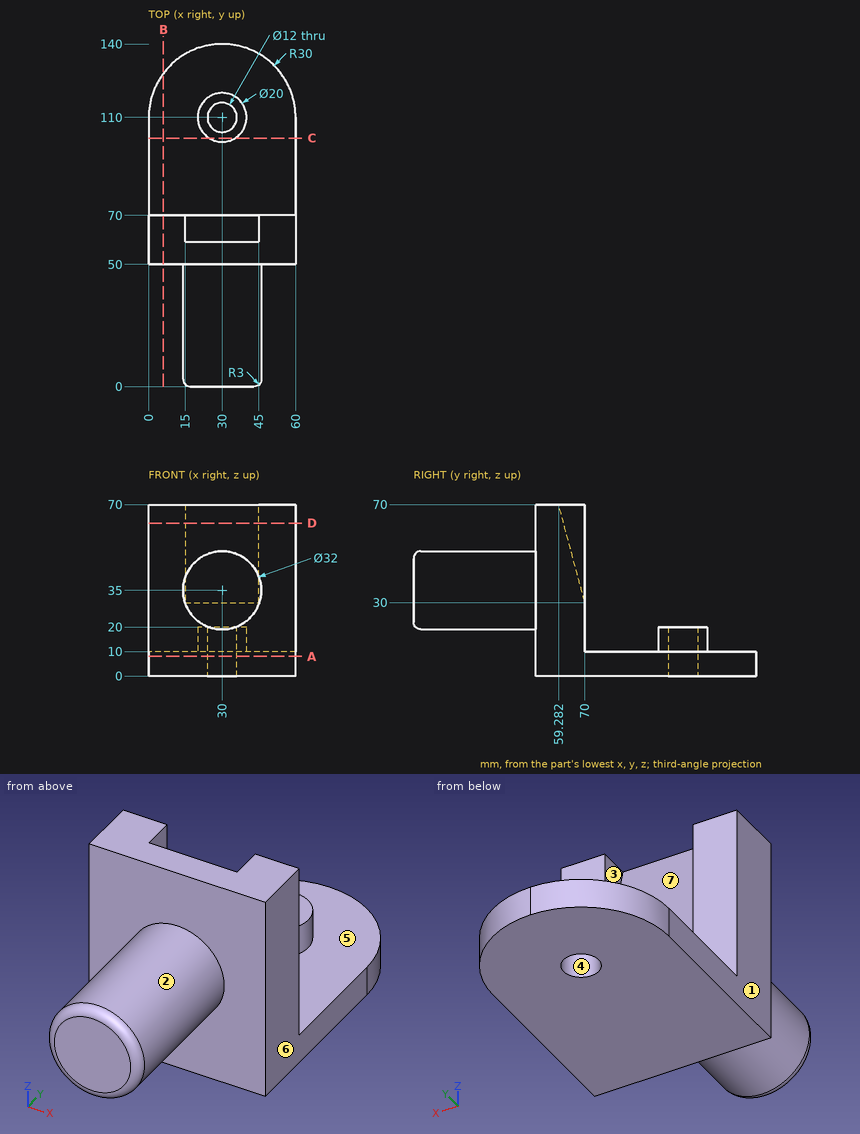
Drawing for the job (mm, zero at the part's lowest x, y, z). A direction names the side the tool comes from. Round coordinates to 2 decimals unless told otherwise and drop trailing zeros. Loops run counter-clockwise (first coordinate to the right, second up) from the corner with the lowest first, then second, coordinate; pieces in that order, holes last.
1. Tool access for the marked faces 1, 2 and 3: list every direction of +Z, -Z, +X, -X, +Y, -Y with a clear straight run to the whole face (end or side of a thin tool).
Check values:
face 1: +Z, -Z, -X, +Y, -Y
face 2: -Y
face 3: +Z, +Y
2. Band-saw the part on C-C, the plane y = 101.5. List the corners of the cut face in (x, z), and give its area (3 significant figures).
Check values:
outline: (0, 0) - (60, 0) - (60, 10) - (35.27, 10) - (35.27, 20) - (24.73, 20) - (24.73, 10) - (0, 10) - close
area: 705 mm2
3. Wall check: probe 1 along Y at (x, z) = (30, 15); probe 2 along Z at (x, y) = (3, 87.5); probe 3 along Z at (x, y) = (31.5, 118.5). Give the ranges that are in metal, low to high.
Check values:
probe 1: y = 50 to 70, 100 to 104, 116 to 120
probe 2: z = 0 to 10
probe 3: z = 0 to 20
4. Band-saw the part on B-B, the plane x = 6. List the corners of the cut face in (y, z), and give its area (3 significant figures).
Check values:
outline: (50, 0) - (128, 0) - (128, 10) - (70, 10) - (70, 70) - (50, 70) - close
area: 1,980 mm2
5. Band-saw the part on D-D, the plane z = 62.5. List the corners of the cut face in (x, y).
Check values:
outline: (0, 50) - (60, 50) - (60, 70) - (45, 70) - (45, 61.29) - (15, 61.29) - (15, 70) - (0, 70) - close
6. Band-saw the part on A-A, the plane z = 8. List the corners of the cut face in (x, y), and give its area (3 significant figures).
Check values:
outline: (0, 50) - (60, 50) - (60, 110) arc R30 ccw to (30, 140) arc R30 ccw to (0, 110) - close; hole circle Ø12 at (30, 110)
area: 4,900 mm2
7. Drop flat-ended pins along their axis: P1, Ø1, axis at x = 30.5, z = 57.5, coming from the +Y side; P2, Ø2, axis at x = 14, z = 60.5, coming from the +Y side; P3, Ø16, axis at x = 29, y = 108.5, coming from the +Z side; P4, Ø9.5, axis at x = 30, y = 110, coming from the +Z side. Give the stop position or say it passes through.
Check values:
P1: stops at y = 62.77
P2: stops at y = 70
P3: stops at z = 20
P4: passes through
8. Mould opens along X. For the marked faces 4, 5, 6 and 7 say: +X half, -X half, draft (parallel to the pull), parting line (faces both ways), or undercut.
Check values:
face 4: undercut
face 5: draft
face 6: +X half
face 7: undercut
